Can you work these out from the model? Positions are in its coordinate system, mm. Face numbers are marked on the shaded views. A direction names the side the tool comes from. Give positions to 0.01 mm unless a question says otherwise; leave off trailing zeros. Write each loop counter-clockwise with the first axis right and the second up, starting at its lowest first coordinate (ties: lowest second). Pieces come first, ordered by that corner, then holes.
from build123d import *

# Parameters (mm, degrees)
F1_DEPTH = 25.4
F2_W     = 6.35
F2_H     = 12.7
F3_DEPTH = 6.35
F4_W     = 7.0131157884
F4_H     = 12.7
F5_DEPTH = 12.7


# Not quite as in the source:
# - a feature names something its author has since deleted; it is built from what else it names


with BuildPart() as f1:
    # F0 (on Front) → F1 (new body)
    with BuildSketch(Plane.XZ):
        Polygon((6.35, 25.4), (0, 25.4), (0, 0), (38.1, 0), (38.1, 12.7), (6.35, 12.7), align=None)
    extrude(amount=F1_DEPTH)

    # F2 (on face) → F3 (cut)
    with BuildSketch(Plane.XY.offset(25.4)):
        with Locations((3.175, -12.7)):
            Rectangle(F2_W, F2_H)
    extrude(amount=-F3_DEPTH, mode=Mode.SUBTRACT)

    # F4 (on face) → F5 (cut)
    with BuildSketch(Plane.XY.offset(12.7)):
        with Locations((34.5934421058, -12.7)):
            Rectangle(F4_W, F4_H)
    extrude(amount=-F5_DEPTH, mode=Mode.SUBTRACT)


solid = f1.part
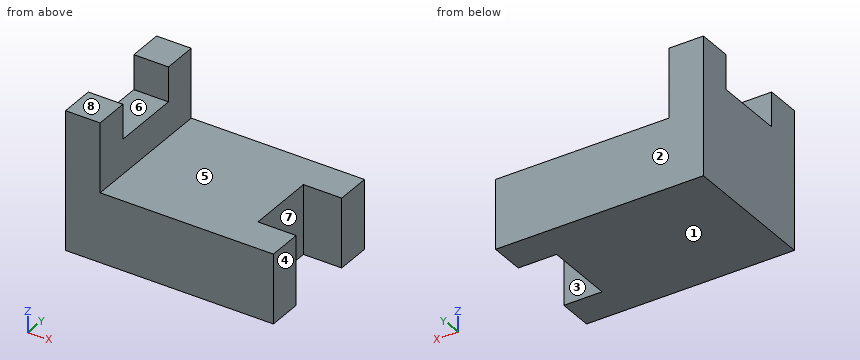
(1) If we mould it in two halves opening along Y, with no side actions, what happens to the marked faces 1, 2 and 3? For each: +Y half, -Y half, draft (parallel to the pull), parting line (faces both ways), or undercut.
Returned:
face 1: draft
face 2: +Y half
face 3: undercut
(2) Will these pins go through, and if not, where does the flat tip stop? P1, Ø12, axis at x = 31, z = 6, coming from the +Y side; P2, Ø10, axis at y = -12, z = 9.5, coming from the +X side; P3, Ø5, axis at x = 2, y = -13, coming from the +Z side; P4, Ø7.5, axis at x = 14.5, y = -11, coming from the +Z side.
Returned:
P1: stops at y = 0
P2: stops at x = 31.09
P3: stops at z = 19.05
P4: stops at z = 12.7
(3) Imagine slicing it at A-A, the plane z = 21.5. Write out the boundary of the cut face in (x, y), plus the area to 3 significant figures.
Returned:
outline: (0, -25.4) - (6.35, -25.4) - (6.35, -19.05) - (0, -19.05) - close; (0, -6.35) - (6.35, -6.35) - (6.35, 0) - (0, 0) - close
area: 80.6 mm2
(4) Imagine slicing it at D-D, the plane x = 9. Write out the boundary of the cut face in (y, z).
Returned:
outline: (-25.4, 0) - (0, 0) - (0, 12.7) - (-25.4, 12.7) - close
(5) Imagine slicing it at B-B, the plane y = -5. Write out the boundary of the cut face in (x, z).
Returned:
outline: (0, 0) - (38.1, 0) - (38.1, 12.7) - (6.35, 12.7) - (6.35, 25.4) - (0, 25.4) - close
(6) For the marked faces 4, 5, 6, 7 and 8, which set-ups out of +Z, -Z, +X, -X, +Y, -Y let a thin tool reach every point of the face, with its end or its side?
Returned:
face 4: +Z, -Z, +X, +Y, -Y
face 5: +Z, +X, +Y, -Y
face 6: +Z, +X, -X
face 7: +Z, -Z, +X
face 8: +Z, +X, -X, +Y, -Y
(7) If I drill on L1, parallel to Z at x = 17, y = -17.75; L2, parallel to Z at x = 3.5, y = -19; L3, parallel to X at y = -14.75, z = 6.25, over which ranges is the centre line in solid material (lowest first)?
Returned:
L1: z = 0 to 12.7
L2: z = 0 to 19.05
L3: x = 0 to 31.09
(8) Imagine slicing it at C-C, the plane z = 5.5. Write out the boundary of the cut face in (x, y).
Returned:
outline: (0, -25.4) - (38.1, -25.4) - (38.1, -19.05) - (31.09, -19.05) - (31.09, -6.35) - (38.1, -6.35) - (38.1, 0) - (0, 0) - close
